Design review of the part built by this model. Coordinates are the model's own, in mm. Coordinates: 2 decimals unless noted, no trailing zeros. Loops run counter-clockwise (first coordinate to the right, second up) from the corner with the lowest first, then second, coordinate; pieces in that order, holes last.
Q1. For P1, Ø2, axis at x = 149, y = 1, coming from the +Z side, flat-tipped, find the tip position at first contact; note if it passes through.
Q2. Wall thickness on probe 1 along Z at (x, y) = (177.8, 2.25); probe 2 along Z at (x, y) = (1, 5); probe 3 along X at (y, z) = (3, 25.4): over which ranges is each line inside the solid? List them lowest first.
Q3. Add section D-D on x = -5.5. Give the boundary of the cut face in (y, z).
Q4. Add section A-A on x = 127. Give the boundary of the cut face in (y, z), and give its area (3 significant figures).
Q5. Add section B-B on x = 177.8. Give the boundary of the cut face in (y, z).
Q6. Add section C-C on y = 1.75. Give the number of separate pieces and of enclosed holes in the cut face, and give its area (3 significant figures).
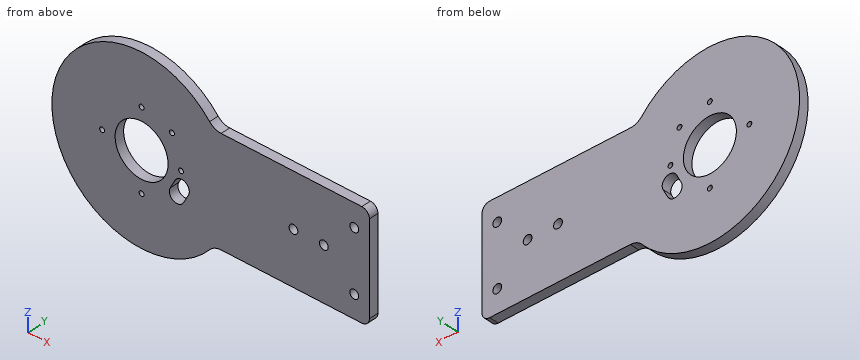
```python
from build123d import *

# Parameters (mm, degrees)
BOSS_EXTRUDE1_DEPTH     = 7.9375
SKETCH23_R              = 22.1615
SKETCH23_R_2            = 2.0193
CUT_EXTRUDE4_DEPTH      = 205.886363401
L_0_29_DIAMETER_HOLE1_D = 7.366
FILLET2_R               = 6.35
FILLET3_R               = 12.7


with BuildPart() as part:
    # Sketch1 → Boss-Extrude1 (new body)
    with BuildSketch(Plane(origin=(0, 0, 0), x_dir=(1, 0, 0), z_dir=(0, 1, 0))):
        with BuildLine():
            Line((190.5, -44.45), (60.409978491, -44.45))
            ThreePointArc((60.409978491, -44.45), (-75.00112, 0), (60.409978491, 44.45))
            Line((60.409978491, 44.45), (190.5, 44.45))
            Line((190.5, 44.45), (190.5, -44.45))
        make_face()
    extrude(amount=BOSS_EXTRUDE1_DEPTH)

    # Sketch23 → Cut-Extrude4 (cut, through all)
    with BuildSketch(Plane.XZ):
        with Locations(Location((0, 0, 0), (0, 0, 270))):
            Circle(SKETCH23_R)
        with Locations(Location((0, 33.02, 0), (0, 0, 270))):
            Circle(SKETCH23_R_2)
        with Locations(Location((33.02, 0, 0), (0, 0, 270))):
            Circle(SKETCH23_R_2)
        with Locations(Location((0, -33.02, 0), (0, 0, 270))):
            Circle(SKETCH23_R_2)
        with Locations(Location((-33.02, 0, 0), (0, 0, 270))):
            Circle(SKETCH23_R_2)
        with Locations(Location((25.4, 25.4, 0), (0, 0, 270))):
            Circle(SKETCH23_R_2)
        with BuildLine():
            Line((23.915755925, -17.31778977), (27.903416949, -9.657564215))
            ThreePointArc((27.903416949, -9.657564215), (36.468039434, -6.957149118), (39.16845453, -15.521771603))
            Line((39.16845453, -15.521771603), (35.180793507, -23.181997158))
            ThreePointArc((35.180793507, -23.181997158), (26.616171022, -25.882412255), (23.915755925, -17.31778977))
        make_face()
    extrude(amount=-CUT_EXTRUDE4_DEPTH, mode=Mode.SUBTRACT)

    # L (0.29) Diameter Hole1 (through all)
    with Locations(Plane(origin=(0, 7.9375, 0), x_dir=(1, 0, 0), z_dir=(0, 1, 0))):
        with Locations((177.8, 25.4), (177.8, -25.4), (152.4, 0), (127, 0)):
            Hole(L_0_29_DIAMETER_HOLE1_D / 2)

    # Fillet2
    fillet2_edges = [part.edges().sort_by_distance(p)[0] for p in [
        (190.5, 3.96875, -44.45),
        (190.5, 3.96875, 44.45),
    ]]
    fillet(fillet2_edges, radius=FILLET2_R)

    # Fillet3
    fillet3_edges = [part.edges().sort_by_distance(p)[0] for p in [
        (60.409978491, 3.96875, -44.45),
        (60.409978491, 3.96875, 44.45),
    ]]
    fillet(fillet3_edges, radius=FILLET3_R)


solid = part.part
```
Entries:
1. P1: stops at z = 44.45
2. probe 1: z = -44.45 to -29.08, -21.72 to 21.72, 29.08 to 44.45
2. probe 2: z = -74.99 to -34.77, -31.27 to -22.14, 22.14 to 31.27, 34.77 to 74.99
2. probe 3: x = -70.57 to 23.38, 27.42 to 174.12, 181.48 to 190.5
3. outline: (0, -74.8) - (7.94, -74.8) - (7.94, -21.47) - (0, -21.47) - close; (0, 21.47) - (7.94, 21.47) - (7.94, 74.8) - (0, 74.8) - close
4. outline: (0, -44.45) - (7.94, -44.45) - (7.94, -3.68) - (0, -3.68) - close; (0, 3.68) - (7.94, 3.68) - (7.94, 44.45) - (0, 44.45) - close
4. area: 647 mm2
5. outline: (0, -44.45) - (7.94, -44.45) - (7.94, -29.08) - (0, -29.08) - close; (0, -21.72) - (7.94, -21.72) - (7.94, 21.72) - (0, 21.72) - close; (0, 29.08) - (7.94, 29.08) - (7.94, 44.45) - (0, 44.45) - close
6. separate pieces: 1
6. enclosed holes: 11
6. area: 26,300 mm2
